Here's how the part is built. I have some questions about the finished solid (model axes, mm). A direction names the side the tool comes from. Round coordinates to 2 decimals unless told otherwise and drop trailing zeros. Write each loop counter-clockwise with the first axis right and the second up, starting at its lowest first coordinate (ties: lowest second). Pieces come first, ordered by that corner, then holes. Notation, with made-up numbers: (3.25, 51.5) - (28.25, 51.5) arc R29 ccw to (28.25, 75.5) - close; hole circle Ø2 at (-5.5, 66). An arc over 180 degrees is marked (long way). One line per question, with ' | ' between items. Start each with the question number.
(1) Thinking about a two-plate mould opening in Y: for faces 3 (the flat face through (0, 1, -19.05)), 4 (the flat face through (0, 23, -2.395)), 5 (the flat face through (0, 88.9, 0)), 6 (the cylindrical face through (0.056, -63.176, 0.876)), which applies, pulls with the +Y half, pulls with the -Y half, needs draft (parallel to the pull), parting line crosses it, or undercut?
(2) Imagine slicing it at B-B (z = 0). Write out the boundary of the cut face in (x, y).
(3) If I drill on L1, parallel to Y at x = -0.5, z = 0; L2, parallel to Z at x = 0.75, y = -69.85; L3, parallel to Y at x = -0.5, z = -8, over which ranges is the centre line in solid material (lowest first)?
(4) Imagine slicing it at D-D (y = 66). Write out the boundary of the cut face in (x, z).
(5) Imagine slicing it at A-A (y = -69.85). Write out the boundary of the cut face in (x, z).
(6) Imagine slicing it at C-C (x = 2). Write out the boundary of the cut face in (y, z), plus the area to 3 significant figures.
(7) For faces 1 (the flat face through (0, 1, 19.05)), 2 (the flat face through (0, 19.253, -7)), which set-ups out of +Z, -Z, +X, -X, +Y, -Y let a thin tool reach every point of the face, with its end or its side?
from build123d import *

# Parameters (mm, degrees)
SKETCH1_W               = 7.9375
SKETCH1_H               = 177.8
EXTRUDE_THIN1_DEPTH     = 19.05
SKETCH2_R               = 6.731
CUT_EXTRUDE1_DEPTH      = 4.96875
CUT_EXTRUDE1_DEPTH_BACK = 5.08
SKETCH3_W               = 8.382
SKETCH3_H               = 6.858
CUT_EXTRUDE2_DEPTH      = 4.96875
CUT_EXTRUDE2_DEPTH_BACK = 4.96875


with BuildPart() as part:
    # Sketch1 → Extrude-Thin1 (new body, symmetric)
    with BuildSketch(Plane.XY):
        Rectangle(SKETCH1_W, SKETCH1_H)
    extrude(amount=EXTRUDE_THIN1_DEPTH, both=True)

    # Sketch2 → Cut-Extrude1 (cut, two sides)
    with BuildSketch(Plane(origin=(0, 0, 0), x_dir=(0, 0, -1), z_dir=(1, 0, 0))) as cut_extrude1_sk:
        with Locations((0, 69.85)):
            Circle(SKETCH2_R)
        with Locations((0, -69.85)):
            Circle(SKETCH2_R)
    extrude(amount=CUT_EXTRUDE1_DEPTH, mode=Mode.SUBTRACT)
    extrude(cut_extrude1_sk.sketch, amount=-CUT_EXTRUDE1_DEPTH_BACK, mode=Mode.SUBTRACT)

    # Sketch3 → Cut-Extrude2 (cut, two sides)
    with BuildSketch(Plane(origin=(0, 0, 0), x_dir=(0, 0, -1), z_dir=(1, 0, 0))) as cut_extrude2_sk:
        with Locations((6.58622, 22.6822)):
            Rectangle(SKETCH3_W, SKETCH3_H)
    extrude(amount=CUT_EXTRUDE2_DEPTH, mode=Mode.SUBTRACT)
    extrude(cut_extrude2_sk.sketch, amount=-CUT_EXTRUDE2_DEPTH_BACK, mode=Mode.SUBTRACT)


solid = part.part
Check sheet entries:
1) face 3: needs draft | face 4: undercut | face 5: pulls with the +Y half | face 6: undercut
2) outline: (-3.97, -88.9) - (3.97, -88.9) - (3.97, -76.58) - (-3.97, -76.58) - close; (-3.97, -63.12) - (3.97, -63.12) - (3.97, 63.12) - (-3.97, 63.12) - close; (-3.97, 76.58) - (3.97, 76.58) - (3.97, 88.9) - (-3.97, 88.9) - close
3) L1: -88.9 to -76.58, -63.12 to 63.12, 76.58 to 88.9 | L2: -19.05 to -6.73, 6.73 to 19.05 | L3: -88.9 to 19.25, 26.11 to 88.9
4) outline: (-3.97, -19.05) - (3.97, -19.05) - (3.97, -5.52) - (-3.97, -5.52) - close; (-3.97, 5.52) - (3.97, 5.52) - (3.97, 19.05) - (-3.97, 19.05) - close
5) outline: (-3.97, -19.05) - (3.97, -19.05) - (3.97, -6.73) - (-3.97, -6.73) - close; (-3.97, 6.73) - (3.97, 6.73) - (3.97, 19.05) - (-3.97, 19.05) - close
6) outline: (-88.9, -19.05) - (88.9, -19.05) - (88.9, 19.05) - (-88.9, 19.05) - close; hole circle Ø13.46 at (-69.85, 0); hole (19.25, -10.78) - (26.11, -10.78) - (26.11, -2.4) - (19.25, -2.4) - close; hole circle Ø13.46 at (69.85, 0) | area: 6,430 mm^2
7) face 1: +Z, +X, -X, +Y, -Y | face 2: +X, -X
